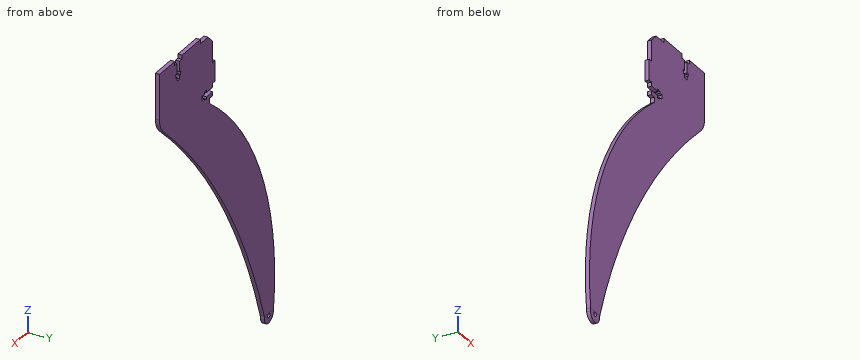
from build123d import *

# Parameters (mm, degrees)
BOSS_EXTRUDE1_DEPTH = 4
SKETCH3_W           = 15
SKETCH3_H           = 4
BOSS_EXTRUDE2_DEPTH = 10
BOSS_EXTRUDE2_TAPER = 2.5
FILLET1_R           = 7.378514
SKETCH4_R           = 2
CUT_EXTRUDE1_DEPTH  = 341.626738097
CUT_EXTRUDE2_DEPTH  = 10
CHAMFER1_SIZE       = 7.5


with BuildPart() as part:
    # Sketch1 → Boss-Extrude1 (new body)
    with BuildSketch(Plane(origin=(0, 0, 0), x_dir=(1, 0, 0), z_dir=(0, 1, 0))):
        with BuildLine():
            Line((87, 0), (87, -4))
            Line((87, -4), (62, -4))
            Line((62, -4), (62, 0))
            Line((62, 0), (50, 0))
            Line((50, 0), (50, -4))
            Line((50, -4), (20, -4))
            Line((20, -4), (20, 0))
            Line((20, 0), (0, 0))
            Line((0, 0), (0, 28))
            Line((0, 28), (-4, 28))
            Line((-4, 28), (-4, 48))
            Line((-4, 48), (0, 48))
            Line((0, 48), (0, 60))
            Line((0, 60), (5, 60))
            Line((5, 60), (5, 65))
            ThreePointArc((5, 65), (-80.454718631, 176.159018175), (-100, 315))
            Line((-100, 315), (-85, 315))
            ThreePointArc((-85, 315), (-19.238758626, 174.034445441), (80.549564864, 54.710856263))
            ThreePointArc((80.549564864, 54.710856263), (85.316540302, 48.031460101), (87, 40))
            Line((87, 40), (87, 0))
        make_face()
    extrude(amount=BOSS_EXTRUDE1_DEPTH)

    # Sketch3 → Boss-Extrude2 (add)
    with BuildSketch(Plane(origin=(0, 0, -315), x_dir=(-1, 0, 0), z_dir=(0, 0, -1))):
        with Locations((92.5, 2)):
            Rectangle(SKETCH3_W, SKETCH3_H)
    extrude(amount=BOSS_EXTRUDE2_DEPTH, taper=BOSS_EXTRUDE2_TAPER)

    # Fillet1
    fillet1_edges = [part.edges().sort_by_distance(p)[0] for p in [
        (-85.436609429, 2, -325),
        (-99.563390571, 2, -325),
    ]]
    fillet(fillet1_edges, radius=FILLET1_R - 0.0001)  # a hair under: the kernel refuses the full size

    # Sketch4 → Cut-Extrude1 (cut, through all)
    with BuildSketch(Plane(origin=(0, 4, 0), x_dir=(1, 0, 0), z_dir=(0, 1, 0))):
        with Locations(Location((-92.5, 317.621485949, 0), (0, 0, 270))):
            Circle(SKETCH4_R)
    extrude(amount=-CUT_EXTRUDE1_DEPTH, mode=Mode.SUBTRACT)

    # Sketch5 → Cut-Extrude2 (cut)
    with BuildSketch(Plane(origin=(0, 4, 0), x_dir=(1, 0, 0), z_dir=(0, 1, 0))):
        Polygon((53.9, 10), (53.9, 0), (58.1, 0), (58.1, 10), (60.5, 10), (60.5, 11), (59.75, 11), (59.75, 13.5), (58.1, 13.5), (58.1, 17), (53.9, 17), (53.9, 13.5), (52.25, 13.5), (52.25, 11), (51.5, 11), (51.5, 10), align=None)
        Polygon((10, 56.1), (0, 56.1), (0, 51.9), (10, 51.9), (10, 49.5), (11, 49.5), (11, 50.25), (13.5, 50.25), (13.5, 51.9), (17, 51.9), (17, 56.1), (13.5, 56.1), (13.5, 57.75), (11, 57.75), (11, 58.5), (10, 58.5), align=None)
    extrude(amount=-CUT_EXTRUDE2_DEPTH, mode=Mode.SUBTRACT)

    # Chamfer1
    chamfer1_edges = [part.edges().sort_by_distance(p)[0] for p in [
        (0, 2, 0),
    ]]
    chamfer(chamfer1_edges, length=CHAMFER1_SIZE)


solid = part.part
Verification items for the finished model (mm, model axes). Give positions to 0.01 mm unless a question says otherwise; leave off trailing zeros. Write each loop counter-clockwise with the first axis right and the second up, starting at its lowest first coordinate (ties: lowest second). Pieces come first, ordered by that corner, then holes.
(1) Cross-section at B-B (x = -74). Enter the section's corners in (y, z), plus the area to 3 significant figures.
(2) Cross-section at A-A (z = -35.5). Enter the section's corners in (x, y).
(3) Gauge pin test, flat ends, axial feed: pin 1 (1.3 mm diameter, centred on x = 59, y = 1, fed in from +Z); pin 2 (1.2 mm diameter, centred on x = 52.5, y = 2.5, fed in from -Z); pin 3 (1.2 mm diameter, centred on x = 55.5, y = 2.5, fed in from +Z). Record the tip position at first contact, or that the pin passes through.
(4) Material ranges on line 1 (X direction, y = 2.7, z = -35); line 2 (Z direction, x = 15, y = 0.5); line 3 (X direction, y = 1.05, z = -22.5), recorded low to high.
Worked out:
1. outline: (0, -283.34) - (4, -283.34) - (4, -161.94) - (0, -161.94) - close
1. area: 486 mm2
2. outline: (-4, 0) - (87, 0) - (87, 4) - (-4, 4) - close
3. pin 1: stops at z = 0
3. pin 2: stops at z = -82.93
3. pin 3: stops at z = -17
4. line 1: x = -4 to 87
4. line 2: z = -125.66 to -56.1, -51.9 to 0
4. line 3: x = 0 to 87
